Read the model definition and answer for the solid it produces. Units are mm, in the model's axes. Give positions to 0.01 mm unless a question says otherwise; leave off trailing zeros. Order: outer loops, then holes, each group sorted by start corner. A loop starts at its lowest first (then second) coordinate and runs counter-clockwise, first axis right, second up. Notation, with made-up numbers: (59.25, 43) -> (86.25, 43) arc R19 cw to (86.25, 62) -> close; hole circle Ø6 at (30, 73). An arc over 180 degrees is marked (long way). Use one line per item in the form item = value.
```python
from build123d import *

# Parameters (mm, degrees)
AUFSATZ_LINEAR_AUSTRAGEN1_DEPTH = 3
SCHNITT_LINEAR_AUSTRAGEN1_REACH = 5
SKIZZE2_R                       = 1.5


with BuildPart() as part:
    # Skizze1 → Aufsatz-Linear austragen1 (new body)
    with BuildSketch(Plane.XY):
        with BuildLine():
            Line((-15, -35), (15, -35))
            ThreePointArc((15, -35), (29.142135624, -29.142135624), (35, -15))
            Line((35, -15), (35, 15))
            ThreePointArc((35, 15), (29.142135624, 29.142135624), (15, 35))
            Line((15, 35), (-15, 35))
            ThreePointArc((-15, 35), (-29.142135624, 29.142135624), (-35, 15))
            Line((-35, 15), (-35, -15))
            ThreePointArc((-35, -15), (-29.142135624, -29.142135624), (-15, -35))
        make_face()
    extrude(amount=AUFSATZ_LINEAR_AUSTRAGEN1_DEPTH)

    # Skizze2 → Schnitt-Linear austragen1 (cut, up to next)
    with BuildSketch(Plane.XY.offset(3), mode=Mode.PRIVATE) as schnitt_linear_austragen1_sk1:
        with Locations((-10, 10)):
            Circle(SKIZZE2_R)
    schnitt_linear_austragen1_tool1 = extrude(schnitt_linear_austragen1_sk1.sketch, amount=-SCHNITT_LINEAR_AUSTRAGEN1_REACH, mode=Mode.PRIVATE) & part.part
    add(schnitt_linear_austragen1_tool1.solids().sort_by_distance((-10, 10, 3))[0], mode=Mode.SUBTRACT)
    # Skizze2 → Schnitt-Linear austragen1 (cut, up to next)
    with BuildSketch(Plane.XY.offset(3), mode=Mode.PRIVATE) as schnitt_linear_austragen1_sk2:
        with Locations((10, 10)):
            Circle(SKIZZE2_R)
    schnitt_linear_austragen1_tool2 = extrude(schnitt_linear_austragen1_sk2.sketch, amount=-SCHNITT_LINEAR_AUSTRAGEN1_REACH, mode=Mode.PRIVATE) & part.part
    add(schnitt_linear_austragen1_tool2.solids().sort_by_distance((10, 10, 3))[0], mode=Mode.SUBTRACT)
    # Skizze2 → Schnitt-Linear austragen1 (cut, up to next)
    with BuildSketch(Plane.XY.offset(3), mode=Mode.PRIVATE) as schnitt_linear_austragen1_sk3:
        with Locations((10, -10)):
            Circle(SKIZZE2_R)
    schnitt_linear_austragen1_tool3 = extrude(schnitt_linear_austragen1_sk3.sketch, amount=-SCHNITT_LINEAR_AUSTRAGEN1_REACH, mode=Mode.PRIVATE) & part.part
    add(schnitt_linear_austragen1_tool3.solids().sort_by_distance((10, -10, 3))[0], mode=Mode.SUBTRACT)
    # Skizze2 → Schnitt-Linear austragen1 (cut, up to next)
    with BuildSketch(Plane.XY.offset(3), mode=Mode.PRIVATE) as schnitt_linear_austragen1_sk4:
        with Locations((-10, -10)):
            Circle(SKIZZE2_R)
    schnitt_linear_austragen1_tool4 = extrude(schnitt_linear_austragen1_sk4.sketch, amount=-SCHNITT_LINEAR_AUSTRAGEN1_REACH, mode=Mode.PRIVATE) & part.part
    add(schnitt_linear_austragen1_tool4.solids().sort_by_distance((-10, -10, 3))[0], mode=Mode.SUBTRACT)


solid = part.part
```
Item 1: The part is cut by section A-A on y = -10. Give the vertices of the cut face in (x, z), and give its area (3 significant figures).
Checks:
outline = (-35, 0) -> (-11.5, 0) -> (-11.5, 3) -> (-35, 3) -> close; (-8.5, 0) -> (8.5, 0) -> (8.5, 3) -> (-8.5, 3) -> close; (11.5, 0) -> (35, 0) -> (35, 3) -> (11.5, 3) -> close
area = 192 mm²
Item 2: The part is cut by section C-C on z = 1.95. Give the vertices of the cut face in (x, y).
Checks:
outline = (-35, -15) arc R20 ccw to (-15, -35) -> (15, -35) arc R20 ccw to (35, -15) -> (35, 15) arc R20 ccw to (15, 35) -> (-15, 35) arc R20 ccw to (-35, 15) -> close; hole circle Ø3 at (-10, -10); hole circle Ø3 at (-10, 10); hole circle Ø3 at (10, -10); hole circle Ø3 at (10, 10)
Item 3: The part is cut by section D-D on y = -27. Give the vertices of the cut face in (x, z).
Checks:
outline = (-31, 0) -> (31, 0) -> (31, 3) -> (-31, 3) -> close
Item 4: Straight lines are drawn through the part: L1, parallel to Y at x = -10, z = 1.25; L2, parallel to X at y = 9, z = 2.8; L3, parallel to Y at x = 15.5, z = 2.85. For each, find the intervals that lie inside material, in ascending order. Write a range as from..to.
Checks:
L1 = -35..-11.5, -8.5..8.5, 11.5..35
L2 = -35..-11.12, -8.88..8.88, 11.12..35
L3 = -34.99..34.99
Item 5: Determine the mould class of faces 1 (the flat face through (0, 35, 1)), 2 (the cylindrical face through (-11.2, 9.1, 1.5)), 3 (the flat face through (0, -35, 1)), 4 (the flat face through (0, 0, 0)) for opening direction Y: +Y half, -Y half, draft (parallel to the pull), parting line (faces both ways), or undercut.
Checks:
face_1 = +Y half
face_2 = undercut
face_3 = -Y half
face_4 = draft
Item 6: Given pin 1 Ø2.5 at (x, y) = (-10, -10) entering from -Z; pin 2 Ø6 at (x, y) = (18.5, -23) entering from -Z, each flat-ended and moving along its own axis, determine where each tip first touches the part or whether it passes through.
Checks:
pin_1 = through
pin_2 = 0
